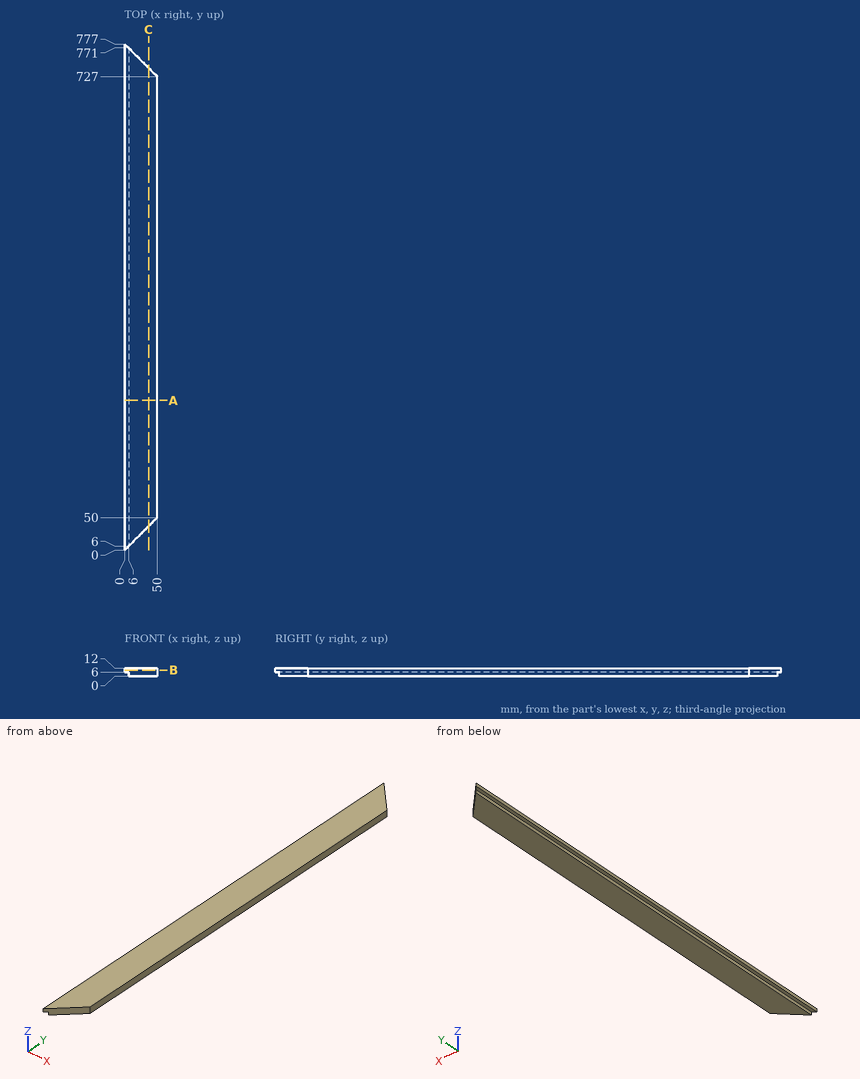
Here's the drawing with two shaded views (mm, measured from the low corner). I have some questions. Coordinates: 2 decimals unless noted, no trailing zeros. Write each loop counter-clockwise with the first axis right and the second up, starting at its lowest first coordinate (ties: lowest second). Pieces come first, ordered by that corner, then holes. Notation, with made-up numbers: M 62.5,13 L 68.5,13 A14 cw 68.5,31 Z; hole C 36.25,57.25 d3. An arc over 180 degrees is marked long. Answer as CSV lines item,"result". Start each with the question number.
1) I want a section at B-B, the plane z = 9. Please give me the cut outline in (x, y), and give its area (4 significant figures).
2) For P1, Ø6.5, axis at x = 4.5, y = 378, coming from the -Z side, with a flat end and sliding along its axis, tell me the tip position at first contact or that it passes through.
3) I want a section at A-A, the plane y = 230. Please give me the cut outline in (x, z).
4) I want a section at C-C, the plane x = 37. Please give me the cut outline in (y, z).
5) Please list where these lines run through material, in increasing order: line 1 (X direction, y = 113, z = 3.5); line 2 (Y direction, x = 47, z = 9.25); line 3 (Y direction, x = 32.5, z = 5.75). Write a range as from..to.
Data:
1,outline,"M 0,0 L 50,50 L 50,727 L 0,777 Z"
1,area,"36,350 mm^2"
2,P1,"stops at z = 0"
3,outline,"M 0,6 L 6,6 L 6,0 L 50,0 L 50,12 L 0,12 Z"
4,outline,"M 37,0 L 740,0 L 740,12 L 37,12 Z"
5,line 1,"x = 6..50"
5,line 2,"y = 47..730"
5,line 3,"y = 32.5..744.5"
